The listing builds one solid part. Answer for the finished solid, in the listing's coordinates (mm). Face numbers are marked on the shaded views. A direction names the side the tool comes from. Round coordinates to 2 decimals unless told otherwise and drop trailing zeros. Write each loop counter-clockwise with the first axis right and the second up, starting at its lowest first coordinate (ties: lowest second). Pieces come first, ordered by that corner, then holes.
(1) A cutting plane is placed at A-A, the plane x = 0. Give the vertices of the cut face in (y, z), and give its area (3 significant figures).
(2) The mould has two halves that part along Y. Classify the marked faces 4, 5 and 6: +Y half, -Y half, draft (parallel to the pull), parting line (faces both ways), or undercut.
(3) Each of these flat-tipped pins is pushed along its axis until it touches: pin 1 Ø2.5 at (x, z) = (11.5, 34) entering from -Y; pin 2 Ø3 at (x, z) = (-11.5, 34) entering from -Y; pin 3 Ø1.9 at (x, z) = (11.5, 34) entering from -Y. Where does it stop, or does it pass through?
(4) Find the intervals of material crossed by probe 1 along X at (y, z) = (22, 34); probe 2 along X at (y, z) = (24, 3); probe 3 along Y at (x, z) = (-11.5, 5.5), in increasing order.
(5) A cutting plane is placed at B-B, the plane y = 13. Give the vertices of the cut face in (x, z).
(6) For the marked faces 1, 2 and 3, determine the directions among +Z, -Z, +X, -X, +Y, -Y from which every point of the face is accessible in a straight line to the end or side of a thin tool.
Autodesk Inventor part; units mm, degrees
ref_plane "YZ Plane" through (0, 0, 0) normal (1, 0, 0) x (0, 1, 0)
ref_plane "XZ Plane" through (0, 0, 0) normal (0, 1, 0) x (-1, 0, 0)
ref_plane "XY Plane" through (0, 0, 0) normal (0, 0, 1) x (1, 0, 0)
sketch "Sketch1" plane through (0, 0, 0) normal (0, 0, 1) x (1, 0, 0)
  line L0 (-17.5, 30) -> (17.5, 30)
  line L1 (17.5, 30) -> (17.5, -30)
  line L2 (17.5, -30) -> (-17.5, -30)
  line L3 (-17.5, -30) -> (-17.5, 30)
  line L4 (0, 9.3667) -> (0, 0)
  line L5 (0, 0) -> (7.7585, 0)
  dimension "d0" = 35
  dimension "d1" = 60
extrude "Extrusion1" add sketch "Sketch1" along normal blind 40
sketch "Sketch2" plane through (0, 0, 40) normal (0, 0, 1) x (1, 0, 0)
  arc A0 (-10, 0) -> (10, 0) centre (0, 0) ccw
  line L0 (-17.5, -30) -> (17.5, -30)
  line L1 (-10, 0) -> (-10, 2.5)
  line L2 (-10, 2.5) -> (10, 2.5)
  line L3 (10, 2.5) -> (10, 0)
  dimension "d8" = 2.5
  dimension "d9" = 20
  dimension "d80" = 10
extrude "Extrusion2" cut sketch "Sketch2" against normal up to surface (40 mm away)
fillet "Fillet1" radius 2.5 2 edges at (-10, 2.5, 20) (10, 2.5, 20)
sketch "Sketch6" plane through (-17.5, -30, 0) normal (0, -1, 0) x (1, 0, 0)
  line L0 (17.5, 0) -> (17.5, 25.5492)
  line L1 (0, 0) -> (0, 40) construction
  line L2 (0, 40) -> (35, 40)
  line L3 (35, 0) -> (35, 40)
  point P0 (6, 34)
  point P1 (29, 34)
  dimension "d139" = 6
  dimension "d140" = 6
  dimension "d164" = 6
  dimension "d165" = 6
hole "Hole4" at (-11.5, -30, 34) at (11.5, -30, 34) direction (0, 1, 0) diameter 3.242 depth 12 tip angle 118
mirror "Spiegeln3" about plane through (0, 0, 0) normal (0, 1, 0) of "Hole4"
fillet "Rundung2" radius 2 8 edges at (17.5, 30, 20) (0, 30, 40) (17.5, 0, 40) (-17.5, 30, 20) (17.5, -30, 20) (-17.5, -30, 20) (0, -30, 40) (-17.5, 0, 40)
sketch "Skizze23" plane through (-15.5, 30, 0) normal (0, 1, 0) x (1, 0, 0)
  circle A0 centre (15.5, -19) radius 9.1
  line L0 (0, -40) -> (31, -40)
  line L1 (-2, 0) -> (-2, -38)
  point P0 (15.5, 0)
  dimension "d173" = 18.2
  dimension "d174" = 21
  dimension "d175" = 17.5
extrude "Extrusion14" cut sketch "Skizze23" against normal up to surface
chamfer "Fase1" distance 1 angle 45 14 edges at (-9.1, 30, 19) (0, -10, 0) (9.2679, 1.7679, 0) (0, 2.5, 0) (-9.2679, 1.7679, 0) (0, -10, 40) (-9.2679, 1.7679, 40) (0, 2.5, 40) (9.2679, 1.7679, 40) (0, 2.5, 9.9) (0, 2.5, 28.1) (8.7024, 2.1921, 16.3395) (8.7024, 2.1921, 21.6605) (-9.1, 1.9212, 18.9844)
sketch "Skizze25" plane through (0, 0, 0) normal (0, 0, -1) x (-1, 0, 0)
  line L0 (-17.5, -28) -> (-17.5, 28)
  line L1 (15.5, -30) -> (-15.5, -30)
  line L2 (17.5, 28) -> (17.5, -28)
  line L3 (-15.5, 30) -> (15.5, 30)
  point P0 (0, 0)
  point P1 (-11.5, -24)
  point P2 (-11.5, 24)
  point P3 (11.5, 24)
  point P4 (11.5, -24)
  dimension "d191" = 6
  dimension "d192" = 6
  dimension "d193" = 6
  dimension "d194" = 6
hole "Bohrung5" at (11.5, -24, 0) at (11.5, 24, 0) at (-11.5, 24, 0) at (-11.5, -24, 0) direction (0, 0, 1) diameter 2.459 depth 8.8 tip angle 118
properties part number "103.003.01_Gehaeuse_Granulatfuehrung" material "Polypropylen"
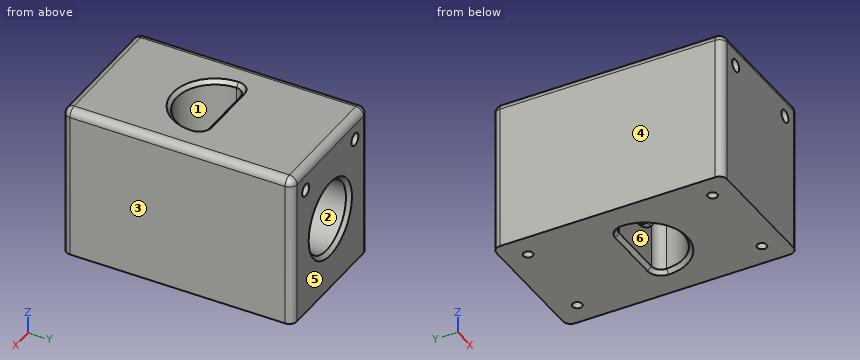
Solutions:
1. outline: (-30, 0) - (-11, 0) - (-10, 1) - (-10, 39) - (-11, 40) - (-28, 40) arc R2 ccw to (-30, 38) - close; (2.5, 1) - (3.5, 0) - (30, 0) - (30, 8.9) - (29, 9.9) - (3.5, 9.9) - (2.5, 8.9) - close; (2.5, 29.1) - (3.5, 28.1) - (29, 28.1) - (30, 29.1) - (30, 38) arc R2 ccw to (28, 40) - (3.5, 40) - (2.5, 39) - close
1. area: 1,390 mm2
2. face 4: draft
2. face 5: +Y half
2. face 6: undercut
3. pin 1: stops at y = -17.78
3. pin 2: stops at y = -17.93
3. pin 3: stops at y = -17.6
4. probe 1: x = -17.5 to -13.12, -9.88 to 9.88, 13.12 to 17.5
4. probe 2: x = -17.5 to -12.73, -10.27 to 10.27, 12.73 to 17.5
4. probe 3: y = -30 to -25.23, -22.77 to 22.77, 25.23 to 30
5. outline: (-17.5, 0) - (17.5, 0) - (17.5, 38) arc R2 ccw to (15.5, 40) - (-15.5, 40) arc R2 ccw to (-17.5, 38) - close; hole circle Ø18.2 at (0, 19)
6. face 1: +Z, -Z
6. face 2: +Y
6. face 3: +Z, -Z, +X, +Y, -Y
